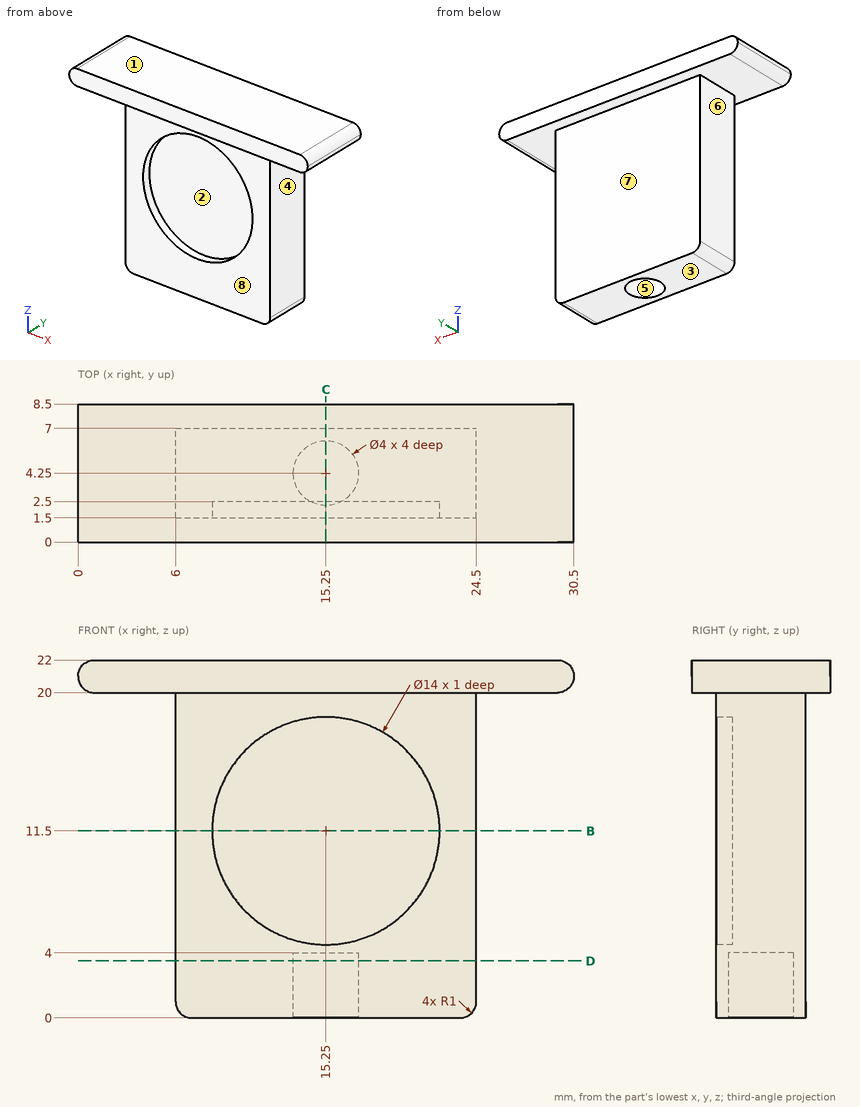
Job drawing, mm, ordinate dimensions from the low corner. One solid piece. A direction names the side the tool comes from. Give positions to 0.01 mm unless a question says otherwise; leave off trailing zeros. Order: outer loops, then holes, each group sorted by start corner. A loop starts at its lowest first (then second) coordinate and runs counter-clockwise, first axis right, second up. Notation, with made-up numbers: (-11.5, 61) - (35.5, 61) arc R13 cw to (35.5, 84) - close; hole circle Ø8 at (73, 15). An arc over 180 degrees is marked (long way). Return JSON: item names as keys, results as strings.
1) Cut at B-B, the plane z = 11.5. Give the cut face in (x, y).
Geometry says:
{"outline": "(6, 1.5) - (8.25, 1.5) - (8.25, 2.5) - (22.25, 2.5) - (22.25, 1.5) - (24.5, 1.5) - (24.5, 7) - (6, 7) - close"}
2) Cut at D-D, the plane z = 3.5. Give the cut face in (x, y).
Geometry says:
{"outline": "(6, 1.5) - (24.5, 1.5) - (24.5, 7) - (6, 7) - close; hole circle Ø4 at (15.25, 4.25)"}
3) Probe line 1 (Z direction, x = 15.25, y = 1.85); line 2 (Y direction, x = 15.25, z = 2.1); line 3 (Y direction, x = 9, z = 15.25). List the from-to ranges inside material, lowest first. Write a range as from..to.
Geometry says:
{"line 1": "0..4.5, 18.5..22", "line 2": "1.5..2.25, 6.25..7", "line 3": "1.5..7"}
4) Pull direction Z, two halves, no side cores. Call the marked faces 1, 2, 3 and 4: pulls with the +Z half, pulls with the -Z half, needs draft (parallel to the pull), parting line crosses it, or undercut.
Geometry says:
{"face 1": "pulls with the +Z half", "face 2": "undercut", "face 3": "pulls with the -Z half", "face 4": "needs draft"}
5) 3-axis set-ups, long thin cutter, end or side, ignore diameter. For the marked faces 5, 6, 7 and 8: which of +Z, -Z, +X, -X, +Y, -Y reach the whole face in a straight line?
Geometry says:
{"face 5": "-Z", "face 6": "-Z, -X, +Y, -Y", "face 7": "-Z, +X, -X, +Y", "face 8": "-Z, +X, -X, -Y"}
6) Cut at C-C, the plane x = 15.25. Give the cut face in (y, z), plus the area to 3 significant figures.
Geometry says:
{"outline": "(0, 20) - (1.5, 20) - (1.5, 18.5) - (2.5, 18.5) - (2.5, 4.5) - (1.5, 4.5) - (1.5, 0) - (2.25, 0) - (2.25, 4) - (6.25, 4) - (6.25, 0) - (7, 0) - (7, 20) - (8.5, 20) - (8.5, 22) - (0, 22) - close", "area": "97.0 mm²"}
7) Flat gauge pins, fed straight in: P1, Ø11, axis at x = 12.5, z = 13, coming from the -Y side; P2, Ø9, axis at x = 11.5, z = 14.5, coming from the +Y side; P3, Ø3, axis at y = 3.5, z = 9.5, coming from the +X side. Where does each tip first touch, or does it go through?
Geometry says:
{"P1": "y = 1.5", "P2": "y = 7", "P3": "x = 24.5"}
